Can you work these out from the model? Positions are in its coordinate system, mm. A direction names the side the tool comes from. Give positions to 0.01 mm unless a question says otherwise; leave off trailing zeros.
from build123d import *

# Parameters (mm, degrees)
BOSS_EXTRUDE1_DEPTH = 19.05
SKETCH2_R           = 1.27
CUT_EXTRUDE1_DEPTH  = 19.05


with BuildPart() as part:
    # Model → Boss-Extrude1 (new body)
    with BuildSketch(Plane.XY):
        with BuildLine():
            Line((152.231072356, -4.329633855), (152.231072356, -8.748222957))
            Line((152.231072356, -8.748222957), (144.734199957, -8.748222957))
            add(Edge.make_bspline(
                [(144.734199957, -8.748222957), (144.69301384, -83.417421729), (84.173632038, -143.939163421), (9.504929576, -143.982778331)],
                knots=[2, 2, 2, 2, 3, 3, 3, 3], degree=3))
            Line((9.504929576, -143.982778331), (9.504929576, -151.455509223))
            Line((9.504929576, -151.455509223), (13.947661262, -151.455509223))
            Line((13.947661262, -151.455509223), (13.947661262, -159.476656261))
            Line((13.947661262, -159.476656261), (9.504930652, -159.476656261))
            Line((9.504930652, -159.476656261), (9.504930652, -167.019727391))
            add(Edge.make_bspline(
                [(9.504930652, -167.019727391), (96.915292045, -167.019727391), (167.775395098, -96.159159251), (167.775412323, -8.748222419)],
                knots=[8, 8, 8, 8, 9, 9, 9, 9], degree=3))
            Line((167.775412323, -8.748222419), (160.207105868, -8.748222419))
            Line((160.207105868, -8.748222419), (160.207105868, -4.329633855))
            Line((160.207105868, -4.329633855), (152.231072356, -4.329633855))
        make_face()
    extrude(amount=BOSS_EXTRUDE1_DEPTH)

    # Sketch2 → Cut-Extrude1 (cut)
    with BuildSketch(Plane.XY.offset(19.05)):
        with Locations((116.443171089, -109.418222003)):
            Circle(SKETCH2_R)
        with Locations((78.695888831, -138.326762479)):
            Circle(SKETCH2_R)
        with Locations((33.680828367, -153.63053201)):
            Circle(SKETCH2_R)
        with Locations((142.586331098, -70.737364147)):
            Circle(SKETCH2_R)
        with Locations((155.238286937, -25.797386475)):
            Circle(SKETCH2_R)
    extrude(amount=-CUT_EXTRUDE1_DEPTH, mode=Mode.SUBTRACT)


solid = part.part
(1) Please list where these lines run through material, in increasing order: probe 1 along Y at (x, z) = (34.5, 2.75); probe 2 along Y at (x, z) = (155, 15.75); probe 3 along X at (y, z) = (-154, 9.25).
Returned:
probe 1: y = -165.06 to -154.6, -152.66 to -141.66
probe 2: y = -71.15 to -27.04, -24.55 to -4.33
probe 3: x = 13.95 to 32.47, 34.9 to 72.47
(2) Which directions (+Z, -Z, +X, -X, +Y, -Y) give clear straight access to the entire face, cutting with the end or side of a thin tool? Please do faces 4 (the flat face through (160.207, -7, 9)), 5 (the flat face through (149, -8.748, 9)), 6 (the flat face through (112, -109, 19.05)), 7 (the flat face through (12, -151.456, 9)), 8 (the flat face through (112, -109, 0)).
Returned:
face 4: +Z, -Z, +X, +Y
face 5: +Z, -Z, -X, +Y
face 6: +Z, +X, -X, +Y, -Y
face 7: +Z, -Z, -X
face 8: -Z, +X, -X, +Y, -Y
(3) Will these pins go through, and if not, where does the flat tip stop? P1, Ø8.5, axis at x = 164.5, z = 11, coming from the +Y side; P2, Ø1.5, axis at x = 33.68, y = -153.63, coming from the +Z side; P3, Ø1.3, axis at y = -7, z = 9.5, coming from the -X side; P4, Ø2.5, axis at y = -155.5, z = 13, coming from the -X side.
Returned:
P1: stops at y = -8.75
P2: passes through
P3: stops at x = 152.23
P4: stops at x = 13.95
(4) Thinking about a two-plate mould opening in Y: for faces 1 (the flat face through (152.231, -7, 9)), 2 (the flat face through (12, -159.477, 9)), 3 (the flat face through (164, -8.748, 9)), which applies, pulls with the +Y half, pulls with the -Y half, needs draft (parallel to the pull), parting line crosses it, or undercut?
Returned:
face 1: needs draft
face 2: undercut
face 3: pulls with the +Y half
(5) Suppose I cut it at A-A on z = 8.25. Give the number of separate pieces and of enclosed holes in the cut face, plus the area to 3 significant figures.
Returned:
separate pieces: 1
enclosed holes: 5
area: 5,290 mm2
